For this review, take the finished solid that the model builds, in its own axes (mm). Face numbers are marked on the shaded views. A direction names the side the tool comes from. Coordinates: 2 decimals unless noted, no trailing zeros. Loops run counter-clockwise (first coordinate to the right, second up) from the corner with the lowest first, then second, coordinate; pieces in that order, holes last.
```python
from build123d import *

# Parameters (mm, degrees)
F2_DEPTH  = 6.35
F5_DEPTH  = 5.08
F5_FACE_W = 12.7
F5_FACE_H = 6.35
F6_DEPTH  = 5.08
F6_TAPER  = 10
F7_R      = 1.27


# Not quite as in the source:
# - a variable given as a bare number and used for a length is read in inches; the dataset says mm whatever the document's units were


with BuildPart() as f2:
    # F1 (on Top) → F2 (new body)
    with BuildSketch(Plane.XY):
        Polygon((-25.4, -23.8125), (-12.7, -23.8125), (-12.7, -17.4625), (-16.7687909609, -17.4625), (-25.4, -17.4625), align=None)
        with BuildLine():
            Line((-12.7, -23.8125), (-4.6920856358, -6.4022057634))
            ThreePointArc((-4.6920856358, -6.4022057634), (-7.6835843575, -1.991591743), (-7.2112720666, 3.3168451022))
            Line((-7.2112720666, 3.3168451022), (-16.7687909609, -17.4625))
            Line((-16.7687909609, -17.4625), (-12.7, -17.4625))
            Line((-12.7, -17.4625), (-12.7, -23.8125))
        make_face()
        with BuildLine():
            ThreePointArc((-1.4422544133, 0.6633690204), (0, 1.5875), (1.4422544133, 0.6633690204))
            Line((1.4422544133, 0.6633690204), (4.6920856358, -6.4022057634))
            ThreePointArc((4.6920856358, -6.4022057634), (7.079807059, -3.5889048828), (7.9375, 0))
            ThreePointArc((7.9375, 0), (7.7538177138, 1.6977093717), (7.2112720666, 3.3168451022))
            ThreePointArc((7.2112720666, 3.3168451022), (0, 7.9375), (-7.2112720666, 3.3168451022))
            ThreePointArc((-7.2112720666, 3.3168451022), (-7.6835843575, -1.991591743), (-4.6920856358, -6.4022057634))
            Line((-4.6920856358, -6.4022057634), (-1.4422544133, 0.6633690204))
        make_face()
        with BuildLine():
            ThreePointArc((7.9375, 0), (7.079807059, -3.5889048828), (4.6920856358, -6.4022057634))
            Line((4.6920856358, -6.4022057634), (12.7, -23.8125))
            Line((12.7, -23.8125), (12.7, -17.4625))
            Line((12.7, -17.4625), (16.7687909609, -17.4625))
            Line((16.7687909609, -17.4625), (7.2112720666, 3.3168451022))
            ThreePointArc((7.2112720666, 3.3168451022), (7.7538177138, 1.6977093717), (7.9375, 0))
        make_face()
        Polygon((12.7, -17.4625), (12.7, -23.8125), (25.4, -23.8125), (25.4, -17.4625), (16.7687909609, -17.4625), align=None)
    extrude(amount=F2_DEPTH)

    # F4 (on face) → F5 (join)
    with BuildSketch(Plane.XY.offset(6.35)):
        Polygon((-12.7, -23.8125), (-12.7, -17.4625), (-16.7687909609, -17.4625), (-25.4, -17.4625), (-25.4, -23.8125), align=None)
        Polygon((25.4, -17.4625), (16.7687909609, -17.4625), (12.7, -17.4625), (12.7, -23.8125), (25.4, -23.8125), align=None)
    extrude(amount=F5_DEPTH)

    # F5_face (on face) → F6 (join)
    with BuildSketch(Plane(origin=(19.05, -20.6375, 11.43), x_dir=(1, 0, 0), z_dir=(0, 0, 1))):
        Rectangle(F5_FACE_W, F5_FACE_H)
        with Locations((-38.1, 0)):
            Rectangle(F5_FACE_W, F5_FACE_H)
    extrude(amount=F6_DEPTH, taper=F6_TAPER)

    # F7
    f7_edges = [f2.edges().sort_by_distance(p)[0] for p in [
        (19.05, -18.358241, 16.51),
        (13.595741, -20.6375, 16.51),
        (19.05, -22.916759, 16.51),
        (24.504259, -20.6375, 16.51),
        (-19.05, -18.358241, 16.51),
        (-13.595741, -20.6375, 16.51),
        (-19.05, -22.916759, 16.51),
        (-24.504259, -20.6375, 16.51),
        (7.071127, -11.574565, 6.35),
        (-11.990032, -7.072827, 6.35),
    ]]
    fillet(f7_edges, radius=F7_R)


solid = f2.part
```
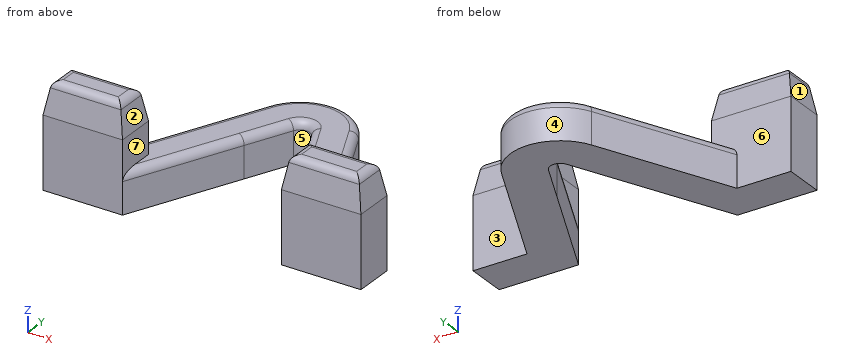
Q1. Consider section C-C (z = 2.75). State the section outline as (x, y) points (1 decimal).
Q2. For pin 1 Ø6 at (y, z) = (-4.5, 5) entering from -X; pin 2 Ø3 at (x, y) = (3.5, -4) entering from +Z; pin 3 Ø9 at (x, z) = (-22, 6) entering from +Y, all flat-tipped, find the tip position at first contact; note any pin that passes through.
Q3. The part is to be moulded in two halves that separate along X. For the marked faces 4, 5, 6 and 7, say which applies: +X half, -X half, draft (parallel to the pull), parting line (faces both ways), or undercut.
Q4. Consider section B-B (x = 17.5). State the section outline as (y, z) points.
Q5. Consider section A-A (z = 8.75). State the section outline as (x, y) points.
Q6. Machinability: for the marked faces 1, 2 and 3, which of the approach directions +Z, -Z, +X, -X, +Y, -Y give a long, thin tool a straight path to every point of the face, cutting with its end or side? Answer none if there is none.
Q7. Wall thickness on probe 1 along X at (y, z) = (-21, 6.75); probe 2 along Y at (x, z) = (13, 7.75); probe 3 along X at (y, z) = (-13.5, 6): over which ranges is each line inside the solid? List them lowest first.
Model answer:
1. outline: (-25.4, -23.8) - (-12.7, -23.8) - (-1.4, 0.7) arc R1.6 cw to (1.4, 0.7) - (12.7, -23.8) - (25.4, -23.8) - (25.4, -17.5) - (16.8, -17.5) - (7.2, 3.3) arc R7.9 ccw to (-7.2, 3.3) - (-16.8, -17.5) - (-25.4, -17.5) - close
2. pin 1: stops at x = -12.19
2. pin 2: stops at z = 6.35
2. pin 3: stops at y = -17.46
3. face 4: parting line
3. face 5: undercut
3. face 6: draft
3. face 7: undercut
4. outline: (-23.81, 0) - (-17.46, 0) - (-17.46, 11.43) - (-18.17, 15.46) arc R1.27 ccw to (-19.42, 16.51) - (-21.85, 16.51) arc R1.27 ccw to (-23.1, 15.46) - (-23.81, 11.43) - close
5. outline: (-25.4, -23.81) - (-12.7, -23.81) - (-12.7, -17.46) - (-25.4, -17.46) - close; (12.7, -23.81) - (25.4, -23.81) - (25.4, -17.46) - (12.7, -17.46) - close
6. face 1: +Z, -X, +Y, -Y
6. face 2: +Z, +Y, -Y
6. face 3: +Z, +X, +Y
7. probe 1: x = -25.4 to -12.7, 12.7 to 25.4
7. probe 2: y = -23.81 to -17.46
7. probe 3: x = -14.51 to -8.39, 8.39 to 14.51
